CAD build for the part. Positions are in the model's coordinates, mm. Face numbers are marked on the shaded views. A direction names the side the tool comes from. Coordinates: 2 decimals unless noted, no trailing zeros. Loops run counter-clockwise (first coordinate to the right, second up) from the corner with the lowest first, then second, coordinate; pieces in that order, holes last. Notation, with made-up numbers: (73.5, 35) -> (115.5, 35) arc R8 cw to (115.5, 50) -> close; hole circle Ø10 at (-27.5, 40.25). An arc over 180 degrees is marked (long way). Answer as CSV lines item,"result". Start each with the question number.
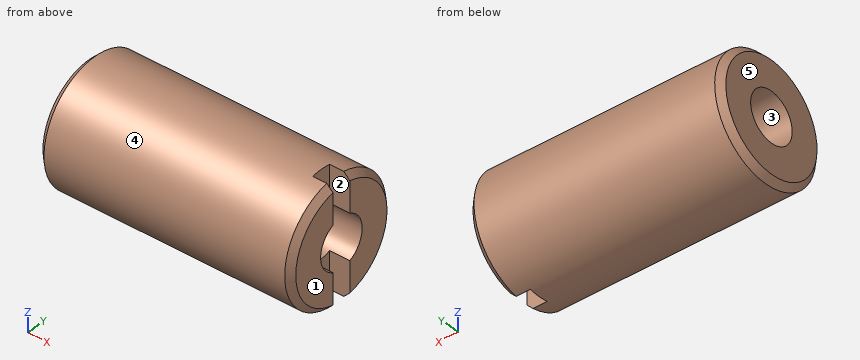
Autodesk Inventor part; units mm, degrees
ref_plane "YZ Plane" through (0, 0, 0) normal (1, 0, 0) x (0, 1, 0)
ref_plane "XZ Plane" through (0, 0, 0) normal (0, 1, 0) x (-1, 0, 0)
ref_plane "XY Plane" through (0, 0, 0) normal (0, 0, 1) x (1, 0, 0)
sketch "スケッチ1" plane through (0, 0, 0) normal (0, 1, 0) x (-1, 0, 0)
  line L0 (0, 0) -> (12.5, 0)
  line L1 (12.5, 0) -> (12.5, -3)
  line L2 (12.5, -3) -> (0, -3)
  line L3 (0, -3) -> (0, 0)
  dimension "d0" = 12.5
  dimension "d1" = 3
revolve "回転1" add sketch "スケッチ1" angle 360 about axis through (0, 0, 0) along (-1, 0, 0)
sketch "スケッチ2" plane through (0, 0, 0) normal (1, 0, 0) x (0, 0, -1)
  point P0 (0, 0)
  point P1 (0, 0)
hole "穴1" at (0, 0, 0) direction (-1, 0, 0) diameter 2.459 end through all
sketch "スケッチ3" plane through (0, 0, 0) normal (1, 0, 0) x (0, 0, -1)
  circle A0 centre (0, 0) radius 3
  line L0 (3, 0) -> (-3, 0)
  line L1 (3, -0.5) -> (-3, -0.5)
  line L2 (3, 0.5) -> (-3, 0.5)
  line L3 (3, 0.5) -> (3, -0.5)
  line L4 (-3, 0.5) -> (-3, -0.5)
  point P0 (-2.958, -0.5)
  point P1 (2.958, -0.5)
  point P2 (2.958, 0.5)
  point P3 (-2.958, 0.5)
  dimension "d10" = 0.5
extrude "押し出し1" cut sketch "スケッチ3" against normal blind 1 contours L0 A0 L2 | A0 L1 L0
chamfer "面取り1" distance 0.3 angle 45 3 edges at (-12.5, 0, 3) (0, 3, 0) (0, -3, 0)
properties part number "BRU-312.5S"
Q1. Pin check, flat tips, straight feed: pin 1 Ø0.8 at (x, z) = (-0.5, -2) entering from -Y; pin 2 Ø1.1 at (y, z) = (0, 2.5) entering from +X; pin 3 Ø1.1 at (x, z) = (-0.5, 2.5) entering from -Y; pin 4 Ø0.8 at (x, z) = (-0.5, -2) entering from +Y. Stop position of each tip, or through.
Q2. Probe probe 1 along Z at (x, y) = (-4.25, 0); probe 2 along Y at (x, z) = (-2.5, 0.5). List the from-to ranges inside material, lowest first. Write a range as from..to.
Q3. Saw through at B-B (y = 0). List the corners of the cut face in (x, z).
Q4. Two-plate mould, pull along Z, no slides. Class the marked faces 3, 4 and 5: pulls with the +Z half, pulls with the -Z half, needs draft (parallel to the pull), parting line crosses it, or undercut.
Q5. Saw through at C-C (x = -3.5). List the corners of the cut face in (y, z).
Q6. Which spindle directions (+Z, -Z, +X, -X, +Y, -Y) get a long thin tool onto all of the face, cutting with end or side? Do the marked faces 1 and 2. Say none if no direction does.
Q7. Saw through at A-A (z = 0). List the corners of the cut face in (x, y), and give its area (3 significant figures).
Ans:
1,pin 1,"stops at y = -2.54"
1,pin 2,"stops at x = 0"
1,pin 3,"stops at y = -2.28"
1,pin 4,"stops at y = 2.54"
2,probe 1,"z = -3..-1.23, 1.23..3"
2,probe 2,"y = -2.96..-1.12, 1.12..2.96"
3,outline,"(-12.5, -2.7) -> (-12.2, -3) -> (-1, -3) -> (-1, -1.23) -> (-12.5, -1.23) -> close; (-12.5, 1.23) -> (-1, 1.23) -> (-1, 3) -> (-12.2, 3) -> (-12.5, 2.7) -> close"
4,face 3,"undercut"
4,face 4,"parting line crosses it"
4,face 5,"needs draft"
5,outline,"circle Ø6 at (0, 0); hole circle Ø2.46 at (0, 0)"
6,face 1,"+Z, -Z, +X, +Y, -Y"
6,face 2,"+Z, -Z, +X"
7,outline,"(-12.5, -2.7) -> (-12.2, -3) -> (-0.3, -3) -> (0, -2.7) -> (0, -1.23) -> (-12.5, -1.23) -> close; (-12.5, 1.23) -> (0, 1.23) -> (0, 2.7) -> (-0.3, 3) -> (-12.2, 3) -> (-12.5, 2.7) -> close"
7,area,"44.1 mm²"
